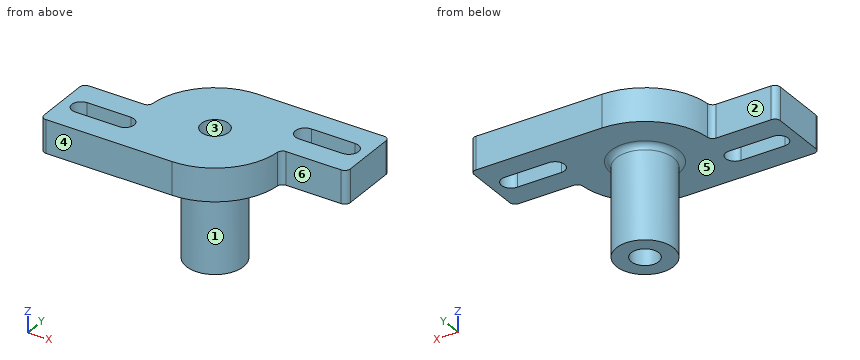
from build123d import *

# Parameters (mm, degrees)
BOSS_EXTRUDE1_DEPTH = 3
SKETCH2_R           = 2.6
BOSS_EXTRUDE2_DEPTH = 8.5
M3_TAPPED_HOLE1_D   = 2.5
FILLET1_R           = 0.5


with BuildPart() as part:
    # Sketch1 → Boss-Extrude1 (new body)
    with BuildSketch(Plane.XY):
        with BuildLine():
            Line((-47.789798407, 94.395653496), (-35.789798407, 94.395653496))
            Line((-35.789798407, 94.395653496), (-35.789798407, 88.395653496))
            Line((-35.789798407, 88.395653496), (-41.789798407, 88.395653496))
            ThreePointArc((-41.789798407, 88.395653496), (-43.54715772, 84.153012809), (-47.789798407, 82.395653496))
            Line((-47.789798407, 82.395653496), (-59.789798407, 82.395653496))
            Line((-59.789798407, 82.395653496), (-59.789798407, 88.395653496))
            Line((-59.789798407, 88.395653496), (-53.789798407, 88.395653496))
            ThreePointArc((-53.789798407, 88.395653496), (-52.032439094, 92.638294183), (-47.789798407, 94.395653496))
        make_face()
        with BuildLine():
            Line((-37.539798407, 90.516657199), (-41.539798407, 90.516657199))
            ThreePointArc((-41.539798407, 90.516657199), (-42.418794704, 91.395653496), (-41.539798407, 92.274649793))
            Line((-41.539798407, 92.274649793), (-37.539798407, 92.274649793))
            ThreePointArc((-37.539798407, 92.274649793), (-36.66080211, 91.395653496), (-37.539798407, 90.516657199))
        make_face(mode=Mode.SUBTRACT)
        with BuildLine():
            Line((-58.039798407, 86.229692735), (-54.039798407, 86.229692735))
            ThreePointArc((-54.039798407, 86.229692735), (-53.205759169, 85.395653496), (-54.039798407, 84.561614258))
            Line((-54.039798407, 84.561614258), (-58.039798407, 84.561614258))
            ThreePointArc((-58.039798407, 84.561614258), (-58.873837646, 85.395653496), (-58.039798407, 86.229692735))
        make_face(mode=Mode.SUBTRACT)
    extrude(amount=BOSS_EXTRUDE1_DEPTH)

    # Sketch2 → Boss-Extrude2 (add)
    with BuildSketch(Plane(origin=(0, 0, 0), x_dir=(-1, 0, 0), z_dir=(0, 0, -1))):
        with Locations(Location((47.789798407, 88.395653496, 0), (0, 0, 180))):
            Circle(SKETCH2_R)
    extrude(amount=BOSS_EXTRUDE2_DEPTH)

    # M3 Tapped Hole1 (through all)
    with Locations(Plane(origin=(0, 0, -8.5), x_dir=(-1, 0, 0), z_dir=(0, 0, -1))):
        with Locations((47.789798407, 88.395653496)):
            Hole(M3_TAPPED_HOLE1_D / 2)

    # Fillet1
    fillet1_edges = [part.edges().sort_by_distance(p)[0] for p in [
        (-35.789798407, 94.395653496, 1.5),
        (-35.789798407, 88.395653496, 1.5),
        (-41.789798407, 88.395653496, 1.5),
        (-59.789798407, 82.395653496, 1.5),
        (-59.789798407, 88.395653496, 1.5),
        (-53.789798407, 88.395653496, 1.5),
        (-50.389798407, 88.395653496, 0),
    ]]
    fillet(fillet1_edges, radius=FILLET1_R)


solid = part.part
Could you check a few things on this model? Use its own coordinates, in mm. Face numbers are marked on the shaded views. A direction names the side the tool comes from. Give positions to 0.01 mm unless a question says otherwise; leave off trailing zeros. Loops run counter-clockwise (first coordinate to the right, second up) from the corner with the lowest first, then second, coordinate; pieces in that order, holes last. Notation, with made-up numbers: (55, -20.5) -> (91, -20.5) arc R20 ccw to (91, 14.5) -> close; hole circle Ø1 at (49, 5.25). An arc over 180 degrees is marked (long way). Return JSON: item names as keys, results as strings.
Item 1: If we section it at D-D on z = -4.75: List the corners of the cut face in (x, y) for me.
Geometry results:
{"outline": "circle Ø5.2 at (-47.79, 88.4); hole circle Ø2.5 at (-47.79, 88.4)"}
Item 2: If we section it at C-C on x = -39: List the corners of the cut face in (y, z) for me.
Geometry results:
{"outline": "(88.4, 0) -> (90.52, 0) -> (90.52, 3) -> (88.4, 3) -> close; (92.27, 0) -> (94.4, 0) -> (94.4, 3) -> (92.27, 3) -> close"}
Item 3: We'd pull the mould along X, two halves only. Please class the marked faces 1, 2 and 3: +X half, -X half, draft (parallel to the pull), parting line (faces both ways), or undercut.
Geometry results:
{"face 1": "parting line", "face 2": "draft", "face 3": "undercut"}
Item 4: I need wall thicknesses on L1, parallel to X at y = 88.5, z = -5.5; L2, parallel to Z at x = -42.25, y = 92.5; L3, parallel to Y at x = -56.75, z = 0.75. Which ranges of each line are inside material? Lowest first, please. Write a range as from..to.
Geometry results:
{"L1": "x = -50.39..-49.04, -46.54..-45.19", "L2": "z = 0..3", "L3": "y = 82.4..84.56, 86.23..88.4"}
Item 5: If we section it at A-A on x = -57.25: List the corners of the cut face in (y, z) for me.
Geometry results:
{"outline": "(82.4, 0) -> (84.56, 0) -> (84.56, 3) -> (82.4, 3) -> close; (86.23, 0) -> (88.4, 0) -> (88.4, 3) -> (86.23, 3) -> close"}
Item 6: Which directions (+Z, -Z, +X, -X, +Y, -Y) give clear straight access to the entire face, cutting with the end or side of a thin tool? Please do the marked faces 4, 5 and 6.
Geometry results:
{"face 4": "+Z, -Z, +X, -X, -Y", "face 5": "-Z", "face 6": "+Z, -Z, +X, -Y"}
Item 7: If we section it at B-B on z = 1.25: List the corners of the cut face in (x, y) for me.
Geometry results:
{"outline": "(-59.79, 82.9) arc R0.5 ccw to (-59.29, 82.4) -> (-47.79, 82.4) arc R6 ccw to (-41.81, 87.93) arc R0.5 cw to (-41.31, 88.4) -> (-36.29, 88.4) arc R0.5 ccw to (-35.79, 88.9) -> (-35.79, 93.9) arc R0.5 ccw to (-36.29, 94.4) -> (-47.79, 94.4) arc R6 ccw to (-53.77, 88.86) arc R0.5 cw to (-54.27, 88.4) -> (-59.29, 88.4) arc R0.5 ccw to (-59.79, 87.9) -> close; hole (-58.04, 84.56) -> (-54.04, 84.56) arc R0.83 ccw to (-54.04, 86.23) -> (-58.04, 86.23) arc R0.83 ccw to start; hole circle Ø2.5 at (-47.79, 88.4); hole (-41.54, 90.52) -> (-37.54, 90.52) arc R0.88 ccw to (-37.54, 92.27) -> (-41.54, 92.27) arc R0.88 ccw to start"}
Item 8: I'm going to push flat-ended pins straight in: pin 1 (6 mm diameter, centred on y = 88, z = -3.5, fed in from +X); pin 2 (1.5 mm diameter, centred on x = -57, z = 1.5, fed in from +Y); pin 3 (2.5 mm diameter, centred on x = -39, z = 1, fed in from -Y). Where does each tip first touch, or does it pass through?
Geometry results:
{"pin 1": "stops at x = -45.19", "pin 2": "stops at y = 88.4", "pin 3": "stops at y = 88.4"}
